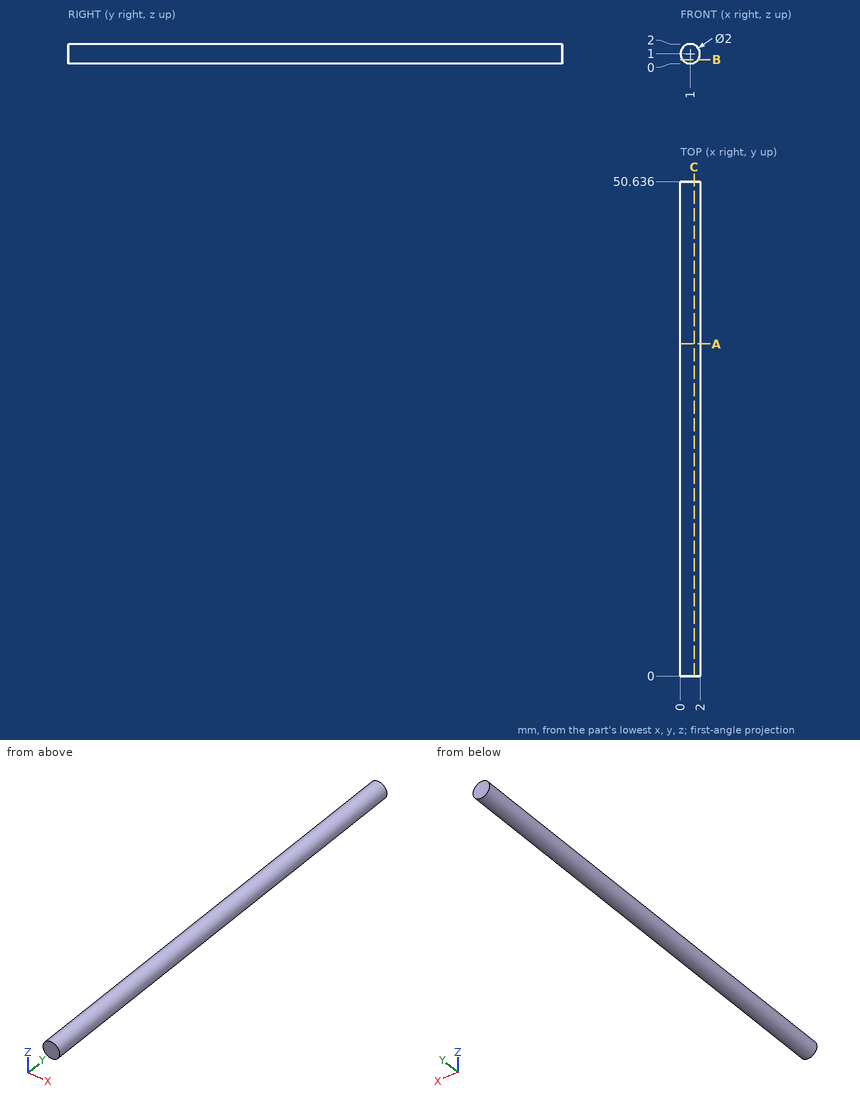
Could you check a few things on this drawing? It's one solid part, dimensions in mm from its lowest x, y, z. Give positions to 0.01 mm unless a question says otherwise; leave off trailing zeros. Order: outer loops, then holes, each group sorted by start corner. A loop starts at its lowest first (then second) coordinate and runs counter-clockwise, first axis right, second up.
1. I need wall thicknesses on L1, parallel to Z at x = 0.9, y = 7; L2, parallel to X at y = 40.5, z = 0.6. Which ranges of each line are inside material? Lowest first, please.
Answers below:
L1: z = 0.01 to 1.99
L2: x = 0.08 to 1.92
2. Suppose I cut it at C-C (x = 1.4). Write out the boundary of the cut face in (y, z), plus the area to 3 significant figures.
Answers below:
outline: (0, 0.08) - (50.64, 0.08) - (50.64, 1.92) - (0, 1.92) - close
area: 92.8 mm2
3. Suppose I cut it at A-A (y = 34). Write out the boundary of the cut face in (x, z), plus the area to 3 significant figures.
Answers below:
outline: circle Ø2 at (1, 1)
area: 3.14 mm2
4. Suppose I cut it at B-B (z = 0.4). Write out the boundary of the cut face in (x, y), plus the area to 3 significant figures.
Answers below:
outline: (0.2, 0) - (1.8, 0) - (1.8, 50.64) - (0.2, 50.64) - close
area: 81.0 mm2
